Source: CAD feature listing. Evaluate the final solid. Frame: model axes, mm. Give positions to 0.01 mm unless a question says otherwise; leave off trailing zeros. Order: outer loops, then holes, each group sorted by start corner. A loop starts at its lowest first (then second) coordinate and runs counter-clockwise, first axis right, second up.
from build123d import *

# Parameters (mm, degrees)
SKETCH1_W           = 80
SKETCH1_H           = 80
BOSS_EXTRUDE1_DEPTH = 3
SKETCH2_R           = 1.75
SKETCH2_R_2         = 2.75
CUT_EXTRUDE1_DEPTH  = 4
SKETCH3_R           = 3.75
CUT_EXTRUDE2_DEPTH  = 4
SKETCH4_R           = 1.25
CUT_EXTRUDE3_DEPTH  = 4
SKETCH5_R           = 2.75
CUT_EXTRUDE4_DEPTH  = 4
SKETCH6_R           = 1.75
CUT_EXTRUDE5_DEPTH  = 4
FILLET1_R           = 2
SKETCH7_R           = 1.75
SKETCH7_R_2         = 2
CUT_EXTRUDE6_DEPTH  = 4


with BuildPart() as part:
    # Sketch1 → Boss-Extrude1 (new body)
    with BuildSketch(Plane(origin=(0, 0, 0), x_dir=(1, 0, 0), z_dir=(0, 1, 0))):
        with Locations((40, 40)):
            Rectangle(SKETCH1_W, SKETCH1_H)
    extrude(amount=BOSS_EXTRUDE1_DEPTH)

    # Sketch2 → Cut-Extrude1 (cut, through all)
    with BuildSketch(Plane(origin=(0, 3, 0), x_dir=(1, 0, 0), z_dir=(0, 1, 0))):
        with Locations((9.29, 40)):
            Circle(SKETCH2_R)
        with Locations((17.33, 40)):
            Circle(SKETCH2_R_2)
    extrude(amount=-CUT_EXTRUDE1_DEPTH, mode=Mode.SUBTRACT)

    # Sketch3 → Cut-Extrude2 (cut, through all)
    with BuildSketch(Plane(origin=(0, 3, 0), x_dir=(1, 0, 0), z_dir=(0, 1, 0))):
        with Locations((61.5, 40)):
            Circle(SKETCH3_R)
    extrude(amount=-CUT_EXTRUDE2_DEPTH, mode=Mode.SUBTRACT)

    # Sketch4 → Cut-Extrude3 (cut, through all)
    with BuildSketch(Plane(origin=(0, 3, 0), x_dir=(1, 0, 0), z_dir=(0, 1, 0))):
        with Locations((66.96, 40)):
            Circle(SKETCH4_R)
        with Locations((56.04, 40)):
            Circle(SKETCH4_R)
        with Locations((61.5, 34.54)):
            Circle(SKETCH4_R)
        with Locations((61.5, 45.46)):
            Circle(SKETCH4_R)
    extrude(amount=-CUT_EXTRUDE3_DEPTH, mode=Mode.SUBTRACT)

    # Sketch5 → Cut-Extrude4 (cut, through all)
    with BuildSketch(Plane(origin=(0, 3, 0), x_dir=(1, 0, 0), z_dir=(0, 1, 0))):
        with Locations((30.25, 40)):
            Circle(SKETCH5_R)
    extrude(amount=-CUT_EXTRUDE4_DEPTH, mode=Mode.SUBTRACT)

    # Sketch6 → Cut-Extrude5 (cut, through all)
    with BuildSketch(Plane(origin=(0, 3, 0), x_dir=(1, 0, 0), z_dir=(0, 1, 0))):
        with Locations((6, 74)):
            Circle(SKETCH6_R)
        with Locations((74, 74)):
            Circle(SKETCH6_R)
        with Locations((74, 6)):
            Circle(SKETCH6_R)
        with Locations((6, 6)):
            Circle(SKETCH6_R)
    extrude(amount=-CUT_EXTRUDE5_DEPTH, mode=Mode.SUBTRACT)

    # Fillet1
    fillet1_edges = [part.edges().sort_by_distance(p)[0] for p in [
        (0, 1.5, -80),
        (80, 1.5, -80),
        (80, 1.5, 0),
        (0, 1.5, 0),
    ]]
    fillet(fillet1_edges, radius=FILLET1_R)

    # Sketch7 → Cut-Extrude6 (cut, through all)
    with BuildSketch(Plane(origin=(0, 3, 0), x_dir=(1, 0, 0), z_dir=(0, 1, 0))):
        with Locations((14, 5)):
            Circle(SKETCH7_R)
        with Locations((66, 5)):
            Circle(SKETCH7_R)
        with Locations((66, 25)):
            Circle(SKETCH7_R)
        with Locations((14, 25)):
            Circle(SKETCH7_R)
        with Locations((14, 75)):
            Circle(SKETCH7_R)
        with Locations((14, 55)):
            Circle(SKETCH7_R)
        with Locations((66, 75)):
            Circle(SKETCH7_R_2)
        with Locations((66, 55)):
            Circle(SKETCH7_R)
    extrude(amount=-CUT_EXTRUDE6_DEPTH, mode=Mode.SUBTRACT)


solid = part.part
1) First-contact query: pin 1 Ø5 at (x, z) = (30.25, -40) entering from -Y; pin 2 Ø4 at (x, z) = (67, -50.5) entering from -Y. Flat tips, straight axial feed; report the tip coordinate or a pass-through.
Checks:
pin 1: passes through
pin 2: stops at y = 0
2) Ray query, L1, parallel to Z at x = 14, y = 0.65; L2, parallel to X at y = 2, z = -34.54; L3, parallel to X at y = 1.5, z = -5. Return the intervals inside material, ascending.
Checks:
L1: z = -80 to -76.75, -73.25 to -56.75, -53.25 to -26.75, -23.25 to -6.75, -3.25 to 0
L2: x = 0 to 60.25, 62.75 to 80
L3: x = 0 to 4.56, 7.44 to 12.25, 15.75 to 64.25, 67.75 to 72.56, 75.44 to 80
3) Section query C-C on y = 1.95. State how many separate pieces and enclosed holes the cut face has, and give its area (3 significant figures).
Checks:
separate pieces: 1
enclosed holes: 20
area: 6,160 mm2
4) Pull-direction query (X, two-part tool) for faces 1 (the face through (67.669, 1.521, -25.526)), 2 (the face through (79.4, 1.52, -79.43)), 3 (the face through (39, 1, -80)); classes: +X half, -X half, draft (parallel to the pull), parting line (faces both ways), or undercut.
Checks:
face 1: undercut
face 2: +X half
face 3: draft
5) Section query D-D on x = 5.5. Output: boundary loops of the cut face in (y, z).
Checks:
outline: (0, -80) - (3, -80) - (3, -75.68) - (0, -75.68) - close; (0, -72.32) - (3, -72.32) - (3, -7.68) - (0, -7.68) - close; (0, -4.32) - (3, -4.32) - (3, 0) - (0, 0) - close
6) Section query B-B on z = -45.46. Output: boundary loops of the cut face in (x, y), and give its area (4 significant figures).
Checks:
outline: (0, 0) - (60.25, 0) - (60.25, 3) - (0, 3) - close; (62.75, 0) - (80, 0) - (80, 3) - (62.75, 3) - close
area: 232.5 mm2
7) Section query A-A on x = 56.04. Output: boundary loops of the cut face in (y, z), and give its area (4 significant figures).
Checks:
outline: (0, -80) - (3, -80) - (3, -41.25) - (0, -41.25) - close; (0, -38.75) - (3, -38.75) - (3, 0) - (0, 0) - close
area: 232.5 mm2
